Autodesk Inventor part; units mm, degrees
ref_plane "YZ Plane" through (0, 0, 0) normal (1, 0, 0) x (0, 1, 0)
ref_plane "XZ Plane" through (0, 0, 0) normal (0, 1, 0) x (-1, 0, 0)
ref_plane "XY Plane" through (0, 0, 0) normal (0, 0, 1) x (1, 0, 0)
ref_plane "작업 평면1" through (0, 0, 0) normal (0, 0, 1) x (1, 0, 0)
ref_plane "작업 평면3" through (0, 0, 6) normal (0, 0, 1) x (1, 0, 0)
ref_plane "작업 평면4" through (40, -20.1, 6) normal (1, 0, 0) x (0, 0, -1)
ref_plane "작업 평면2" through (0, 0, 6) normal (0, 0, 1) x (1, 0, 0)
ref_plane "작업 평면6" through (30, -20.1, 6) normal (1, 0, 0) x (0, 0, -1)
ref_plane "작업 평면5" through (0, 0, 12) normal (0, 0, 1) x (1, 0, 0)
sketch "스케치6" plane through (0, 0, 12) normal (0, 0, 1) x (1, 0, 0)
  arc A0 (0, -7.45) -> (0, 7.45) centre (0, 0) ccw
  arc A1 (0, -7.45) -> (0, -14) centre (0.8514, -10.725) ccw
  line L0 (40, -20.1) -> (0, -14)
  line L1 (40, 20.1) -> (40, -20.1)
  line L2 (0, 14) -> (40, 20.1)
  arc A2 (0, 14) -> (0, 7.45) centre (0.8364, 10.725) ccw
  circle A3 centre (0, -11) radius 1.35
  circle A4 centre (7.7782, -7.7782) radius 1.35
  circle A5 centre (11, 0) radius 1.35
  circle A6 centre (7.7782, 7.7782) radius 1.35
  circle A7 centre (0, 11) radius 1.35
extrude "돌출6" add sketch "스케치6" against normal blind 6
sketch "스케치9" plane through (0, 0, 12) normal (0, 0, 1) x (1, 0, 0)
  arc A0 (0, -7.45) -> (0, 7.45) centre (0, 0) ccw
  arc A1 (0, -7.45) -> (0, -14) centre (0.8514, -10.725) ccw
  line L0 (0, -14) -> (40, -20.1)
  line L1 (40, -20.1) -> (40, 20.1)
  line L2 (40, 20.1) -> (0, 14)
  arc A2 (0, 14) -> (0, 7.45) centre (0.8364, 10.725) ccw
  circle A3 centre (11, 0) radius 1.35
  circle A4 centre (0, 11) radius 1.35
  circle A5 centre (7.7782, 7.7782) radius 1.35
  circle A6 centre (7.7782, -7.7782) radius 1.35
  circle A7 centre (0, -11) radius 1.35
  line L3 (40, 20.1) -> (40, -20.1)
  line L4 (40, -20.1) -> (34, -20.1)
  line L5 (34, -20.1) -> (34, 20.1)
  line L6 (34, 20.1) -> (40, 20.1)
  line L7 (40, 20.1) -> (40, 10.05)
  line L8 (40, 10.05) -> (40, -10.05)
  circle A8 centre (37, 10.05) radius 1.35
  circle A9 centre (37, -10.05) radius 1.35
  dimension "d41" = 6
  dimension "d42" = 10.05
  dimension "d43" = 20.1
  dimension "d44" = 2.7
  dimension "d45" = 2.7
extrude "돌출8" cut sketch "스케치9" against normal blind 6 contours A8 | A9
sketch "스케치10" plane through (0, 0, 12) normal (0, 0, 1) x (1, 0, 0)
  circle A0 centre (37, -10.05) radius 1.35
  circle A1 centre (37, 10.05) radius 1.35
  arc A2 (0, -7.45) -> (0, 7.45) centre (0, 0) ccw
  arc A3 (0, -7.45) -> (0, -14) centre (0.8514, -10.725) ccw
  line L0 (0, -14) -> (40, -20.1)
  line L1 (40, -20.1) -> (40, 20.1)
  line L2 (40, 20.1) -> (0, 14)
  arc A4 (0, 14) -> (0, 7.45) centre (0.8364, 10.725) ccw
  circle A5 centre (11, 0) radius 1.35
  circle A6 centre (0, 11) radius 1.35
  circle A7 centre (7.7782, 7.7782) radius 1.35
  circle A8 centre (7.7782, -7.7782) radius 1.35
  circle A9 centre (0, -11) radius 1.35
  line L3 (34, -5) -> (40, -5)
  line L4 (40, -5) -> (40, 5)
  line L5 (40, 5) -> (34, 5)
  line L6 (34, 5) -> (34, -5)
  line L7 (34, -5) -> (40, 5) construction
  line L8 (40, -5) -> (34, 5) construction
  circle A10 centre (40, 5) radius 0.75
  circle A11 centre (34, 5) radius 0.75
  circle A12 centre (34, -5) radius 0.75
  circle A13 centre (40, -5) radius 0.75
  point P0 (37, 0)
  point P1 (39.25, -5)
  point P2 (40, -5.75)
  point P3 (34, -4.25)
  point P4 (34.75, -5)
  point P5 (34.75, 5)
  point P6 (34, 4.25)
  point P7 (40, 5.75)
  point P8 (39.25, 5)
  dimension "d48" = 10
  dimension "d51" = 1.5
  dimension "d52" = 1.5
  dimension "d53" = 1.5
  dimension "d54" = 1.5
extrude "돌출9" cut sketch "스케치10" against normal blind 10 contours A13 L3 L1 | L1 L5 A10 | L3 A13 L1 | L3 A12 L6 A11 L5 A10 L1 A13 | L1 A10 L5 | A12 L6 L3 | L3 L6 A12 | A11 L6 L5 | L5 L6 A11
properties part number "feet_holder1" material "PMMA 플라스틱"
Check sheet for the modelled part. Datum: model origin and axes. Units: mm. A direction names the side the tool comes from. Give positions to 0.01 mm unless a question says otherwise; leave off trailing zeros. Loops run counter-clockwise (first coordinate to the right, second up) from the corner with the lowest first, then second, coordinate; pieces in that order, holes last. Notation, with made-up numbers: M -37,-9.75 L -13,-9.75 A16 cw -13,-5.75 Z; hole C 77,37.5 d5. An arc over 180 degrees is marked long. Answer as a JSON object with one key per item and string values. Group by question number.
Q1. Cross-section at A-A on x = 4. Record the cut outline in (y, z).
Q2. Release check for a two-part mould opening along X. For faces 3 (the cylindrical face through (33.45, -5.51, 9.04)), 4 (the flat face through (18, 0, 12)), 5 (the flat face through (34, 0, 9)), 6 (the cylindrical face through (6.43, 7.84, 9.04)) record: released by +X, released by -X, zero draft, split by the parting line, or undercut.
Q3. Cross-section at C-C on x = 37. Record the cut outline in (y, z), then the cut area to 3 significant figures.
Q4. Go/stop test with flat-tipped pins: P1, Ø1.5, axis at x = 5.5, z = 7, coming from the +Y side; P2, Ø3, axis at x = 0, y = 11, coming from the +Z side; P3, Ø2, axis at x = 37, z = 9, coming from the -Y side (3 decimals); P4, Ø3.5, axis at x = 37, z = 8.5, coming from the +Y side. Record where each tip stops, or that it passes through.
Q5. Access from +Z, -Z, +X, -X, +Y, -Y to the whole of each face (thin tool, end or side, straight path). Record for faces 1 (the flat face through (37, -5, 9)), 2 (the cylindrical face through (6.78, -6.87, 9.04)).
Q6. Cross-section at D-D on x = 29. Record the cut outline in (y, z).
Q7. Cross-section at B-B on z = 8.4. Record the cut outline in (x, y) (3 decimals), then the cut area to 3 significant figures.
Q8. Material ranges on line 1 along Y through (x, z) = (0, 7.3); line 2 along X through (y, z) = (-10, 6.85); line 3 along X through (y, z) = (12, 8.55), recorded low to high. Write a range as [from, to].
Evaluation:
{
 "1": {"outline": "M -14.61,6 L -6.29,6 L -6.29,12 L -14.61,12 Z; M 6.29,6 L 14.61,6 L 14.61,12 L 6.29,12 Z"},
 "2": {"face 3": "undercut", "face 4": "zero draft", "face 5": "released by +X", "face 6": "undercut"},
 "3": {"outline": "M -19.64,6 L -11.4,6 L -11.4,12 L -19.64,12 Z; M -8.7,6 L -5,6 L -5,12 L -8.7,12 Z; M 5,6 L 8.7,6 L 8.7,12 L 5,12 Z; M 11.4,6 L 19.64,6 L 19.64,12 L 11.4,12 Z", "area": "143 mm2"},
 "4": {"P1": "stops at y = 14.95", "P2": "stops at z = 12", "P3": "stops at y = -19.795", "P4": "stops at y = 19.91"},
 "5": {"face 1": "+Z, -Z, +X", "face 2": "+Z, -Z"},
 "6": {"outline": "M -18.42,6 L 18.42,6 L 18.42,12 L -18.42,12 Z"},
 "7": {"outline": "M 0,-14 L 40,-20.1 L 40,-5.75 A0.75 cw 39.25,-5 L 34.75,-5 A0.75 cw long 34,-4.25 L 34,4.25 A0.75 cw long 34.75,5 L 39.25,5 A0.75 cw 40,5.75 L 40,20.1 L 0,14 A3.38 ccw 0,7.45 A7.45 cw 0,-7.45 A3.384 ccw Z; hole C 0,-11 d2.7; hole C 0,11 d2.7; hole C 7.778,-7.778 d2.7; hole C 7.778,7.778 d2.7; hole C 11,0 d2.7; hole C 37,-10.05 d2.7; hole C 37,10.05 d2.7", "area": "1,200 mm2"},
 "8": {"line 1": "y = [-14, -12.35], [-9.65, -7.45], [7.45, 9.65], [12.35, 14]", "line 2": "x = [-2.45, -0.91], [0.91, 35.65], [38.35, 40]", "line 3": "x = [-2.29, -0.91], [0.91, 40]"}
}
